Autodesk Inventor part; units mm, degrees
ref_plane "YZ Plane" through (0, 0, 0) normal (1, 0, 0) x (0, 1, 0)
ref_plane "XZ Plane" through (0, 0, 0) normal (0, 1, 0) x (-1, 0, 0)
ref_plane "XY Plane" through (0, 0, 0) normal (0, 0, 1) x (1, 0, 0)
sketch "スケッチ1" plane through (0, 0, 0) normal (0, 0, 1) x (1, 0, 0)
  circle A0 centre (0, 0) radius 4
  dimension "d13" = 8
extrude "押し出し1" add sketch "スケッチ1" along normal mid plane 20
sketch "スケッチ2" plane through (0, 0, 10) normal (0, 0, 1) x (1, 0, 0)
  point P0 (0, 0)
  point P1 (0, 0)
hole "穴1" at (0, 0, 10) direction (0, 0, -1) diameter 3.242 depth 11.8 tip angle 118
mirror "ミラー1" about plane through (0, 0, 0) normal (0, 0, 1) of "穴1"
chamfer "面取り1" distance 0.2 angle 45 4 edges at (0, 1.621, 10) (-4, 0, 10) (-4, 0, -10) (0, 1.621, -10)
properties part number "unir-spacer4" material "鋼、炭素鋼"
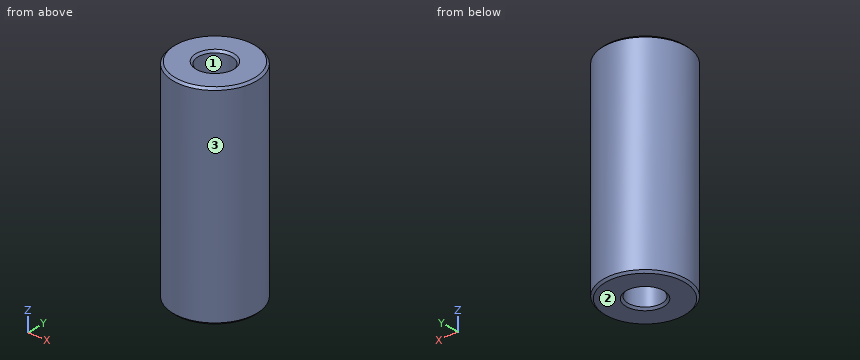
For this review, take the finished solid that the model builds, in its own axes (mm). Face numbers are marked on the shaded views. Coordinates: 2 decimals unless noted, no trailing zeros. Loops run counter-clockwise (first coordinate to the right, second up) from the corner with the lowest first, then second, coordinate; pieces in that order, holes last. Notation, with made-up numbers: (7.25, 23) - (11.25, 23) arc R8 ccw to (11.25, 38) - close; hole circle Ø4 at (69, 81.5). An arc over 180 degrees is marked (long way). Use a Markdown table: item, result. Add a question column.
Item 1: For line 1 (Y direction, x = 0, z = -2.75); line 2 (X direction, y = 0.5, z = 1.5); line 3 (X direction, y = 3.5, z = -2), list the stretches that pass through material, from the lowest coordinate up.
Item 2: We need section A-A (y = 0). Give the boundary of the cut face in (x, z).
Item 3: Mouldability with a two-part tool opening along X and no side actions: class the marked faces 1, 2 and 3 as pulls with the +X half, pulls with the -X half, needs draft (parallel to the pull), parting line crosses it, or undercut.
Item 4: We need section C-C (z = -0.5). Give the boundary of the cut face in (x, y), and give its area (3 significant figures).
Item 5: Insertion check: pin 1 Ø2.5 at (x, y) = (0, 0) entering from -Z; pin 2 Ø1.5 at (x, z) = (1.5, -7.5) entering from -Y; pin 3 Ø1.5 at (x, z) = (-2.5, -7) entering from -Y. Each pin has a flat end and moves straight along its axis. Give the tip position at first contact, or say it passes through.
Results list:
| question | item | result |
|---|---|---|
| 1 | line 1 | y = -4 to -1.62, 1.62 to 4 |
| 1 | line 2 | x = -3.97 to -1.54, 1.54 to 3.97 |
| 1 | line 3 | x = -1.94 to 1.94 |
| 2 | outline | (-4, -9.8) - (-3.8, -10) - (-1.82, -10) - (-1.62, -9.8) - (-1.62, 9.8) - (-1.82, 10) - (-3.8, 10) - (-4, 9.8) - close; (1.62, -9.8) - (1.82, -10) - (3.8, -10) - (4, -9.8) - (4, 9.8) - (3.8, 10) - (1.82, 10) - (1.62, 9.8) - close |
| 3 | face 1 | undercut |
| 3 | face 2 | needs draft |
| 3 | face 3 | parting line crosses it |
| 4 | outline | circle Ø8 at (0, 0); hole circle Ø3.24 at (0, 0) |
| 4 | area | 42.0 mm^2 |
| 5 | pin 1 | passes through |
| 5 | pin 2 | stops at y = -3.93 |
| 5 | pin 3 | stops at y = -3.6 |
